Geometry check sheet. Reference: the model listing, model coordinates, mm. A direction names the side the tool comes from. Coordinates: 2 decimals unless noted, no trailing zeros. Loops run counter-clockwise (first coordinate to the right, second up) from the corner with the lowest first, then second, coordinate; pieces in that order, holes last.
from build123d import *

# Parameters (mm, degrees)
F3_ANGLE = 90
F4_R     = 3
F4_R_2   = 1.7
F5_DEPTH = 0.3
F6_R     = 3
F6_R_2   = 1.7
F7_DEPTH = 0.3


with BuildPart() as f2:
    # F0 (on Front) → F2 (revolve)
    with BuildSketch(Plane.XZ):
        with BuildLine():
            Line((-5, 10), (-5, 1.7))
            Line((-5, 1.7), (5, 1.7))
            Line((5, 1.7), (5, 10))
            Line((5, 10), (1.6867828916, 4.7992908911))
            ThreePointArc((1.6867828916, 4.7992908911), (0, 3.8738901078), (-1.6867828916, 4.7992908911))
            Line((-1.6867828916, 4.7992908911), (-5, 10))
        make_face()
    revolve(axis=Axis((0, 0, 0), (1, 0, 0)))


with BuildPart() as f2_1:
    # F3: moved
    add(f2.part.rotate(Axis((-13.5274957865, 0, 0), (-1, 0, 0)), F3_ANGLE))

    # F4 (on face) → F5 (join)
    with BuildSketch(Plane.YZ.offset(5)):
        Circle(F4_R)
        Circle(F4_R_2, mode=Mode.SUBTRACT)
    extrude(amount=F5_DEPTH)

    # F6 (on face) → F7 (join)
    with BuildSketch(Plane(origin=(-5, 0, 0), x_dir=(0, -1, 0), z_dir=(-1, 0, 0))):
        Circle(F6_R)
        Circle(F6_R_2, mode=Mode.SUBTRACT)
    extrude(amount=F7_DEPTH)


solid = f2_1.part
(1) Access from +Z, -Z, +X, -X, +Y, -Y to the whole of each face (thin tool, end or side, straight path). Record for faces 1 (the cylindrical face through (5.15, -0.65, -2.93)), 2 (the conical face through (-1.894, 4.888, 1.539)), 3 (the flat face through (-5, 2.1, 2.4)).
Findings:
face 1: +X
face 2: none
face 3: -X
(2) Sectioned sample at C-C on x = 1. Record the cut outline in (y, z), and give its area (3 significant figures).
Findings:
outline: circle Ø8.28 at (0, 0); hole circle Ø3.4 at (0, 0)
area: 44.8 mm2
(3) Sectioned sample at A-A on y = 0. Record the cut outline in (x, z).
Findings:
outline: (-5.3, -3) - (-5, -3) - (-5, -10) - (-1.69, -4.8) arc R2 cw to (1.69, -4.8) - (5, -10) - (5, -3) - (5.3, -3) - (5.3, -1.7) - (-5.3, -1.7) - close; (-5.3, 1.7) - (5.3, 1.7) - (5.3, 3) - (5, 3) - (5, 10) - (1.69, 4.8) arc R2 cw to (-1.69, 4.8) - (-5, 10) - (-5, 3) - (-5.3, 3) - close
(4) Draft check along X on faces 4 (the flat face through (5, -2.1, 2.4)), 5 (the conical face through (1.848, -4.009, -3.074)), 6 (the cylindrical face through (-5.15, 0.65, -2.93)). Enter one of: +X half, -X half, draft (parallel to the pull), parting line (faces both ways), or undercut.
Findings:
face 4: +X half
face 5: undercut
face 6: draft
(5) Gauge pin test, flat ends, axial feed: pin 1 Ø2 at (y, z) = (-1, 5) entering from -X; pin 2 Ø1 at (y, z) = (-6.5, 4.5) entering from +X; pin 3 Ø1.5 at (x, z) = (4, 3.5) entering from +Y; pin 4 Ø12 at (y, z) = (-5.5, 5.5) entering from -X. Record the tip position at first contact, or that the pin passes through.
Findings:
pin 1: stops at x = -5
pin 2: stops at x = 5
pin 3: stops at y = 8.98
pin 4: stops at x = -5.3
(6) Scan lines: L1, parallel to Z at x = -5.1, y = 0; L2, parallel to X at y = 6.75, z = -5.25; L3, parallel to X at y = -2.5, z = 4. Record each from-to range of solid material in increasing order.
Findings:
L1: z = -3 to -1.7, 1.7 to 3
L2: x = -5 to -4.08, 4.08 to 5
L3: x = -5 to -1.63, 1.63 to 5
(7) Sectioned sample at D-D on x = -3. Record the cut outline in (y, z).
Findings:
outline: circle Ø13.72 at (0, 0); hole circle Ø3.4 at (0, 0)
